Verification items for this drawing (mm, ordinates from the low corner). Coordinates: 2 decimals unless noted, no trailing zeros. Order: outer loops, then holes, each group sorted by start corner. A loop starts at its lowest first (then second) coordinate and runs counter-clockwise, first axis right, second up. Notation, with made-up numbers: (8.5, -39) -> (39.5, -39) arc R30 ccw to (39.5, -7) -> close; hole circle Ø1 at (80, -21). An arc over 180 degrees is marked (long way). Answer in a Markdown table with one row per item. Add a question column.
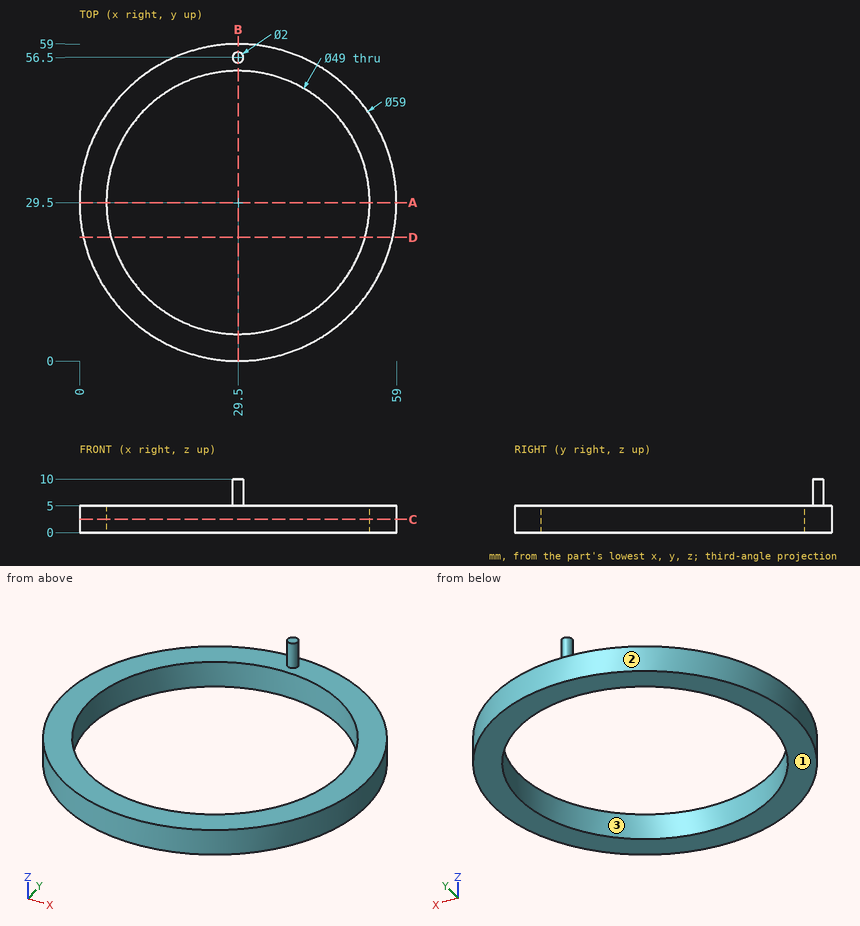
(1) Cross-section at C-C (z = 2.5). Enter the section's corners in (x, y).
(2) Mould release check, pull along X, two halves, no side actions. Record for the marked faces 1, 2 and 3: +X half, -X half, draft (parallel to the pull), parting line (faces both ways), or undercut.
(3) Go/stop test with flat-tipped pins: P1, Ø4, axis at y = 14.5, z = 3, coming from the -X side; P2, Ø6, axis at y = 39.5, z = 6, coming from the +X side (3 decimals). Record where each tip stops, or that it passes through.
(4) Cross-section at D-D (y = 23). Enter the section's corners in (x, z).
(5) Cross-section at B-B (x = 29.5). Enter the section's corners in (y, z), plus the area to 3 significant figures.
(6) Scan lines: line 1 along Y through (x, z) = (29.5, 3.6); line 2 along X through (y, z) = (20, 3.25); line 3 along X through (y, z) = (25.5, 0.5). Record each from-to range of solid material in increasing order.
(7) Cross-section at A-A (y = 29.5). Enter the section's corners in (x, z).
Checks:
| question | item | result |
|---|---|---|
| 1 | outline | circle Ø59 at (29.5, 29.5); hole circle Ø49 at (29.5, 29.5) |
| 2 | face 1 | draft |
| 2 | face 2 | parting line |
| 2 | face 3 | undercut |
| 3 | P1 | x = 3.02 |
| 3 | P2 | x = 58.115 |
| 4 | outline | (0.73, 0) -> (5.88, 0) -> (5.88, 5) -> (0.73, 5) -> close; (53.12, 0) -> (58.27, 0) -> (58.27, 5) -> (53.12, 5) -> close |
| 5 | outline | (0, 0) -> (5, 0) -> (5, 5) -> (0, 5) -> close; (54, 0) -> (59, 0) -> (59, 5) -> (57.5, 5) -> (57.5, 10) -> (55.5, 10) -> (55.5, 5) -> (54, 5) -> close |
| 5 | area | 60.0 mm² |
| 6 | line 1 | 0 to 5, 54 to 59 |
| 6 | line 2 | 1.57 to 6.92, 52.08 to 57.43 |
| 6 | line 3 | 0.27 to 5.33, 53.67 to 58.73 |
| 7 | outline | (0, 0) -> (5, 0) -> (5, 5) -> (0, 5) -> close; (54, 0) -> (59, 0) -> (59, 5) -> (54, 5) -> close |
